The figure shows three views and two pictorial views of one solid part (mm, origin at its lowest corner). Answer the questions. A direction names the side the tool comes from. Round coordinates to 2 decimals unless told otherwise and drop trailing zeros. Order: outer loops, then holes, each group sorted by start corner. A loop starts at its lowest first (then second) coordinate and runs counter-clockwise, first axis right, second up. Notation, with made-up numbers: M 72.25,55.25 L 81.25,55.25 A19 cw 81.25,81.25 Z; hole C 24.5,35.25 d2. An arc over 180 degrees is marked long. Answer as CSV lines item,"result".
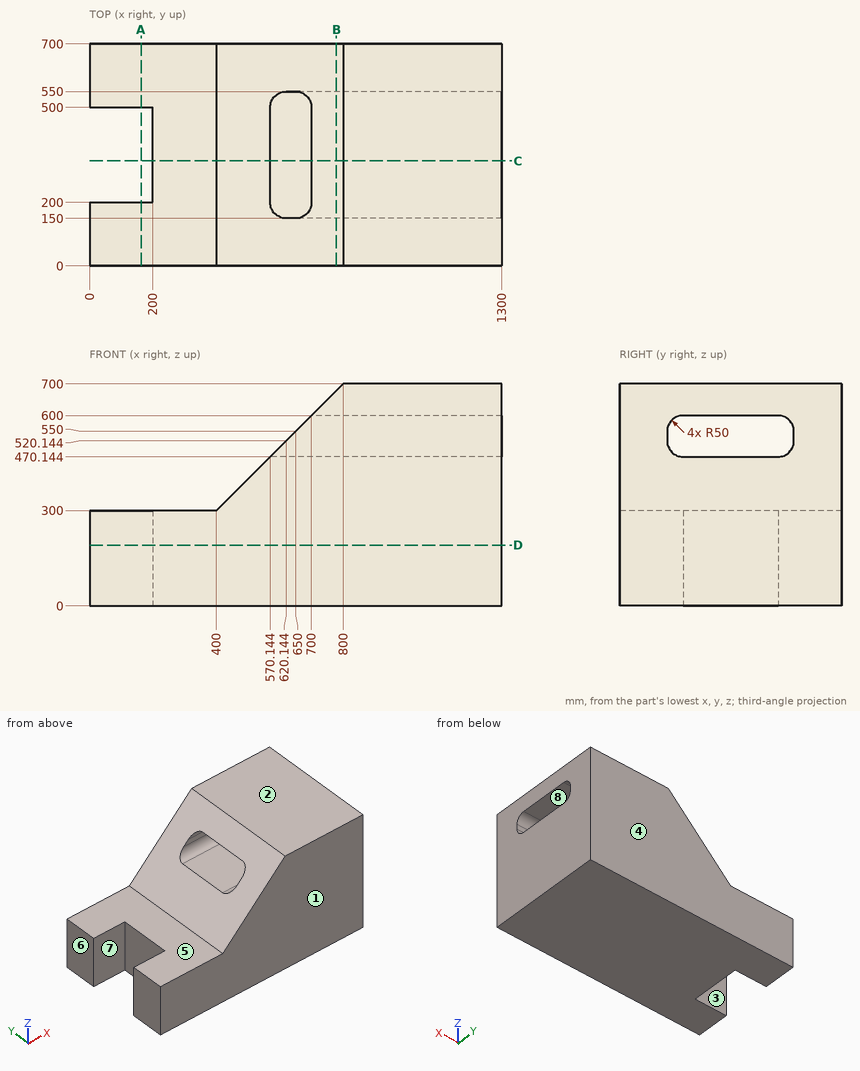
Item 1: Flat-ended cylindrical pins translate along their axes: pin 1 (1.5 mm diameter, centred on x = 680, y = 293.5, fed in from +Z); pin 2 (12 mm diameter, centred on y = 365, z = 105, fed in from -X); pin 3 (6 mm diameter, centred on x = 251, y = 142.5, fed in from +Z). Find the tip coordinate at first contact, or state that the pin passes through.
Ans:
pin 1,"z = 470.14"
pin 2,"x = 200"
pin 3,"z = 300"
Item 2: A cutting plane is placed at C-C, the plane y = 331.5. Determine the outline of the cut face in (x, z).
Ans:
outline,"M 200,0 L 1300,0 L 1300,470.14 L 570.14,470.14 L 400,300 L 200,300 Z; M 700,600 L 1300,600 L 1300,700 L 800,700 Z"
Item 3: A tool of negligible diameter and unlimited length cuts with its end or side. For the marked faces 5, 6, 7 and 8, from which of +Z, -Z, +X, -X, +Y, -Y can it reach the whole face along a straight path? Write none if from no direction.
Ans:
face 5,"+Z, -X, +Y, -Y"
face 6,"+Z, -Z, -X, +Y, -Y"
face 7,"+Z, -Z, -X"
face 8,"+X, -X"
Item 4: A cutting plane is placed at D-D, the plane z = 191. Determine the outline of the cut face in (x, y).
Ans:
outline,"M 0,0 L 1300,0 L 1300,700 L 0,700 L 0,500 L 200,500 L 200,200 L 0,200 Z"
Item 5: Determine the mould class of the marked faces 1, 2, 3 and 4 for opening direction Y: +Y half, -Y half, draft (parallel to the pull), parting line (faces both ways), or undercut.
Ans:
face 1,"-Y half"
face 2,"draft"
face 3,"undercut"
face 4,"+Y half"
Item 6: A cutting plane is placed at B-B, the plane x = 779. Determine the outline of the cut face in (y, z), and give its area (4 significant figures).
Ans:
outline,"M 0,0 L 700,0 L 700,679 L 0,679 Z; hole M 150,520.14 A50 ccw 200,470.14 L 500,470.14 A50 ccw 550,520.14 L 550,550 A50 ccw 500,600 L 200,600 A50 ccw 150,550 Z"
area,"425,500 mm2"
Item 7: A cutting plane is placed at A-A, the plane x = 162.5. Determine the outline of the cut face in (y, z), and give its area (3 significant figures).
Ans:
outline,"M 0,0 L 200,0 L 200,300 L 0,300 Z; M 500,0 L 700,0 L 700,300 L 500,300 Z"
area,"120,000 mm2"
Item 8: Find the intervals of material crossed by probe 1 along Z at (x, y) = (1139, 196); probe 2 along Z at (x, y) = (1238, 286); probe 3 along Y at (x, z) = (1228.5, 526), in increasing order. Write a range as [from, to].
Ans:
probe 1,"[0, 470.3], [599.84, 700]"
probe 2,"[0, 470.14], [600, 700]"
probe 3,"[0, 150], [550, 700]"
